Autodesk Inventor part; units mm, degrees
ref_plane "YZ Plane" through (0, 0, 0) normal (1, 0, 0) x (0, 1, 0)
ref_plane "XZ Plane" through (0, 0, 0) normal (0, 1, 0) x (-1, 0, 0)
ref_plane "XY Plane" through (0, 0, 0) normal (0, 0, 1) x (1, 0, 0)
sketch "Sketch2" plane through (0, 0, 0) normal (0, 0, 1) x (1, 0, 0)
  line L0 (27.4963, -15.875) -> (0, 0) construction
  arc A0 (-38.4948, -9.525) -> (-28.3934, -28.5433) centre (-27.4963, -15.875) ccw
  arc A1 (10.5225, 38.861) -> (-10.9985, 38.1) centre (0, 31.75) ccw
  line L1 (-38.4948, -9.525) -> (-10.9985, 38.1)
  line L2 (10.5225, 38.861) -> (45.7067, -13.2026)
  line L3 (34.2871, -32.9819) -> (-28.3934, -28.5433)
  circle A2 centre (-182.5755, 105.41) radius 190.5 construction
  line L4 (-182.5755, 105.41) -> (0, 0) construction
  line L5 (-133.2704, -78.5989) -> (50.7384, -29.2938) construction
  line L6 (50.7384, -29.2938) -> (1.4334, 154.715) construction
  line L7 (50.7384, -29.2938) -> (0, 0) construction
  arc A3 (34.2871, -32.9819) -> (45.7067, -13.2026) centre (35.1842, -20.3136) ccw
  point P0 (0, 0)
  point P1 (-25.1827, 3.3154)
  point P2 (-20.1512, -15.4625)
  point P3 (-3.3154, -25.1827)
  point P4 (15.4625, -20.1512)
  point P5 (25.1827, -3.3154)
  point P6 (20.1512, 15.4625)
  point P7 (3.3154, 25.1827)
  point P8 (-15.4625, 20.1512)
  dimension "d74" = 31.75
  dimension "d77" = 360
  dimension "d80" = 25.4
  dimension "d83" = 360
  dimension "d96" = 381
  dimension "d97" = 210.82
  dimension "d98" = 12.7
  dimension "d99" = 12.7
  dimension "d100" = 12.7
extrude "Plate2" add sketch "Sketch2" along normal blind 4.7625
hole "Hole3" at (35.1842, -20.3136, 0) at (-27.4963, -15.875, 0) at (0, 31.75, 0) direction (0, 0, 1) diameter 6.5278 end through all
hole "Hole4" at (0, 0, 0) direction (0, 0, 1) diameter 28.575 end through all
hole "Hole5" at (-25.1827, 3.3154, 0) at (15.4625, -20.1512, 0) at (25.1827, -3.3154, 0) at (-15.4625, 20.1512, 0) direction (0, 0, 1) diameter 4.9784 end through all
equation "\"BendRadius\" = Thickness"
equation "\"BendReliefWidth\" = Thickness"
equation "\"BendReliefDepth\" = 0.5 * Thickness"
equation "\"CornerReliefSize\" = 4 * Thickness"
equation "\"MinimumRemnant\" = 2 * Thickness"
equation "\"TransitionRadius\" = BendRadius"
equation "\"JacobiRadiusSize\" = BendRadius"
equation "\"GapSize\" = Thickness"
properties part number "PLATE,TURRET,MOTOR,MOUNT" material "Aluminum 6061"
Could you check a few things on this model? Use its own coordinates, in mm. Give positions to 0.01 mm unless a question says otherwise; leave off trailing zeros. Order: outer loops, then holes, each group sorted by start corner. A loop starts at its lowest first (then second) coordinate and runs counter-clockwise, first axis right, second up.
1. Suppose I cut it at A-A (y = 19.5). List the corners of the cut face in (x, z) for me.
2. We'd pull the mould along X, two halves only. Please class faces 1 (the flat face through (13, -11, 4.762)), 2 (the cylindrical face through (-0.628, -14.274, 2.415)), 3 (the flat face through (3.386, -30.794, 2.348)), 4 (the cylindrical face through (-0.14, 28.49, 2.41)): pulls with the +X half, pulls with the -X half, needs draft (parallel to the pull), parting line crosses it, or undercut.
3. I need wall thicknesses on L1, parallel to X at y = -3, z = 2.15; L2, parallel to X at y = 3, z = 4.6; L3, parallel to Y at x = -8.5, z = 4.35. Which ranges of each line are inside material? Lowest first, please.
4. Suppose I cut it at C-C (y = 3.5). List the corners of the cut face in (x, z) for me, plus the area to 3 significant figures.
5. Suppose I cut it at B-B (x = 7). List the corners of the cut face in (y, z) for me, plus the area to 3 significant figures.
6. Suppose I cut it at D-D (z = 2.7). Give the number of separate pieces and of enclosed holes in the cut face, plus the area to 3 significant figures.
7. Will these pins go through, and if not, where does the flat tip stop? P1, Ø2, axis at y = 32.5, z = 3, coming from the +X side; P2, Ø2, axis at x = 5.5, z = 2, coming from the +Y side; P3, Ø2, axis at y = 21, z = 1, coming from the -X side.
Solved:
1. outline: (-21.74, 0) - (-17.87, 0) - (-17.87, 4.76) - (-21.74, 4.76) - close; (-13.06, 0) - (23.61, 0) - (23.61, 4.76) - (-13.06, 4.76) - close
2. face 1: needs draft
2. face 2: undercut
2. face 3: pulls with the -X half
2. face 4: undercut
3. L1: x = -34.73 to -13.97, 13.97 to 22.71, 27.65 to 38.81
3. L2: x = -31.26 to -27.65, -22.71 to -13.97, 13.97 to 34.76
3. L3: y = -29.95 to -11.48, 11.48 to 41.19
4. outline: (-30.97, 0) - (-27.67, 0) - (-27.67, 4.76) - (-30.97, 4.76) - close; (-22.7, 0) - (-13.85, 0) - (-13.85, 4.76) - (-22.7, 4.76) - close; (13.85, 0) - (34.42, 0) - (34.42, 4.76) - (13.85, 4.76) - close
4. area: 156 mm2
5. outline: (-31.05, 0) - (-12.46, 0) - (-12.46, 4.76) - (-31.05, 4.76) - close; (12.46, 0) - (42.35, 0) - (42.35, 4.76) - (12.46, 4.76) - close
5. area: 231 mm2
6. separate pieces: 1
6. enclosed holes: 8
6. area: 3,540 mm2
7. P1: stops at x = 15.5
7. P2: stops at y = 43.63
7. P3: stops at x = -21.45
